Autodesk Inventor part; units mm, degrees
ref_plane "YZ Plane" through (0, 0, 0) normal (1, 0, 0) x (0, 1, 0)
ref_plane "XZ Plane" through (0, 0, 0) normal (0, 1, 0) x (-1, 0, 0)
ref_plane "XY Plane" through (0, 0, 0) normal (0, 0, 1) x (1, 0, 0)
sketch "Эскиз1" plane through (0, 0, 0) normal (1, 0, 0) x (0, 1, 0)
  line L0 (-20.211, 11.7625) -> (-20.211, 0.7625)
  line L1 (-20.211, 0.7625) -> (-0.211, 0.7625)
  line L2 (-0.211, 0.7625) -> (-0.211, -7.2375)
  line L3 (-0.211, -7.2375) -> (-22.211, -7.2375)
  line L4 (-22.211, -7.2375) -> (-22.211, -22.2375)
  line L5 (-20.211, 11.7625) -> (-50.211, 11.7625)
  line L6 (-50.211, 11.7625) -> (-50.211, 5.7625)
  line L7 (-50.211, 5.7625) -> (-42.211, 5.7625)
  line L8 (-42.211, 5.7625) -> (-42.211, -2.2375)
  line L9 (-42.211, -2.2375) -> (-50.211, -2.2375)
  line L10 (-50.211, -2.2375) -> (-50.211, -10.2375)
  line L11 (-50.211, -10.2375) -> (-38.211, -10.2375)
  line L12 (-38.211, -10.2375) -> (-38.211, -22.2375)
  line L13 (-38.211, -22.2375) -> (-22.211, -22.2375)
  point P0 (0, 0)
  dimension "d0" = 15
  dimension "d1" = 22
  dimension "d2" = 20
  dimension "d3" = 11
  dimension "d4" = 12
  dimension "d5" = 12
  dimension "d6" = 8
  dimension "d7" = 6
  dimension "d8" = 50
  dimension "d9" = 50
  dimension "d10" = 34
  dimension "d11" = 8
sketch "Эскиз2" plane through (0, 0, 0) normal (1, 0, 0) x (0, 1, 0)
  line L0 (-49.3354, 11.5668) -> (-49.3354, 17.5668)
  line L1 (-49.3354, 17.5668) -> (-14.2528, 17.5668)
  point P0 (0, 0)
  dimension "d12" = 6
revolve "Вращение1" add sketch "Эскиз1" angle 360 about axis through (0, -49.3354, 17.5668) along (0, 1, 0)
properties part number "Задание номер 3"
Check sheet for the modelled part. Datum: model origin and axes. Units: mm. A direction names the side the tool comes from. Round coordinates to 2 decimals unless told otherwise and drop trailing zeros. Loops run counter-clockwise (first coordinate to the right, second up) from the corner with the lowest first, then second, coordinate; pieces in that order, holes last. Notation, with made-up numbers: M 7,40 L 36,40 A14 ccw 36,47 Z; hole C -37,48 d11. An arc over 180 degrees is marked long. One line per question, with ' | ' between items. Start each with the question number.
Item 1: Section check A-A (x = 0). Record the boundary of the cut face in (y, z).
Item 2: Section check D-D (y = -5). Record the boundary of the cut face in (x, z).
Item 3: Scan lines: probe 1 along Z at (x, y) = (0, -44); probe 2 along Z at (x, y) = (0, -35.5); probe 3 along Z at (x, y) = (0, -10). Record each from-to range of solid material in increasing order.
Item 4: Section check B-B (z = 2). Record the boundary of the cut face in (x, y).
Item 5: Set-up check for faces 1 (the face through (0.255, -35.421, 23.365)), 2 (the face through (-27, -38.211, 9)), 3 (the face through (0, -20.211, 10)): record each of +Z, -Z, +X, -X, +Y, -Y from which the full face is reachable in a straight line by a thin tool's end or side.
Item 6: Release check for a two-part mould opening along X. For faces 4 (the face through (-39.466, -30.099, 22.749)), 5 (the face through (-6.6, -50.211, 36.5)), 6 (the face through (-7.585, -46.267, -0.727)), 7 (the face through (9, -42.211, 9)) record: released by +X, released by -X, zero draft, split by the parting line, or undercut.
Item 7: Section check C-C (x = 8). Record the boundary of the cut face in (y, z), and give its area (3 significant figures).
Item 8: Gauge pin test, flat ends, axial feed: pin 1 Ø2 at (x, y) = (20.5, -36) entering from -Z; pin 2 Ø2 at (x, y) = (5, -14) entering from -Z; pin 3 Ø2 at (y, z) = (-26.5, 3.5) entering from -X. Record the tip position at first contact, or that the pin passes through.
Worked out:
1) outline: M -50.21,-10.24 L -38.21,-10.24 L -38.21,-22.24 L -22.21,-22.24 L -22.21,-7.24 L -0.21,-7.24 L -0.21,0.76 L -20.21,0.76 L -20.21,11.76 L -50.21,11.76 L -50.21,5.76 L -42.21,5.76 L -42.21,-2.24 L -50.21,-2.24 Z; M -50.21,23.37 L -20.21,23.37 L -20.21,34.37 L -0.21,34.37 L -0.21,42.37 L -22.21,42.37 L -22.21,57.37 L -38.21,57.37 L -38.21,45.37 L -50.21,45.37 L -50.21,37.37 L -42.21,37.37 L -42.21,29.37 L -50.21,29.37 Z
2) outline: C 0,17.57 d49.61; hole C 0,17.57 d33.61
3) probe 1: -10.24 to -2.24, 5.76 to 11.76, 23.37 to 29.37, 37.37 to 45.37 | probe 2: -22.24 to 11.76, 23.37 to 57.37 | probe 3: -7.24 to 0.76, 34.37 to 42.37
4) outline: M -36.63,-38.21 L -23.04,-38.21 L -23.04,-50.21 L -12.24,-50.21 L -12.24,-42.21 L 12.24,-42.21 L 12.24,-50.21 L 23.04,-50.21 L 23.04,-38.21 L 36.63,-38.21 L 36.63,-22.21 L 19.31,-22.21 L 19.31,-0.21 L 6.33,-0.21 L 6.33,-20.21 L -6.33,-20.21 L -6.33,-0.21 L -19.31,-0.21 L -19.31,-22.21 L -36.63,-22.21 Z
5) face 1: +Y, -Y | face 2: -Y | face 3: +Y
6) face 4: split by the parting line | face 5: zero draft | face 6: undercut | face 7: undercut
7) outline: M -50.21,-9.06 L -38.21,-9.06 L -38.21,-21.43 L -22.21,-21.43 L -22.21,-5.91 L -0.21,-5.91 L -0.21,2.79 L -20.21,2.79 L -20.21,32.34 L -0.21,32.34 L -0.21,41.05 L -22.21,41.05 L -22.21,56.56 L -38.21,56.56 L -38.21,44.2 L -50.21,44.2 L -50.21,35.68 L -42.21,35.68 L -42.21,26.25 L -50.21,26.25 L -50.21,8.89 L -42.21,8.89 L -42.21,-0.55 L -50.21,-0.55 Z | area: 2,180 mm^2
8) pin 1: z = -17.13 | pin 2: z = -6.91 | pin 3: x = -37.6
